```python
from build123d import *

# Parameters (mm, degrees)
SKETCH1_W           = 165
SKETCH1_H           = 330
BOSS_EXTRUDE1_DEPTH = 4
SKETCH2_R           = 37.5
CUT_EXTRUDE1_DEPTH  = 202.285866369
SKETCH4_W           = 8
SKETCH4_H           = 300
CUT_EXTRUDE3_DEPTH  = 202.285866369
SKETCH3_W           = 4
SKETCH3_H           = 20
CUT_EXTRUDE2_DEPTH  = 202.285866369
SKETCH5_W           = 8
SKETCH5_H           = 30
CUT_EXTRUDE4_DEPTH  = 202.285866369
SKETCH6_R           = 2
CUT_EXTRUDE5_DEPTH  = 198.838317825
SKETCH7_R           = 2
CUT_EXTRUDE6_DEPTH  = 198.838317825
SKETCH8_W           = 153
SKETCH8_H           = 20
CUT_EXTRUDE7_DEPTH  = 198.838317825


with BuildPart() as part:
    # Sketch1 → Boss-Extrude1 (new body)
    with BuildSketch(Plane.XY):
        with Locations((7.5, -15)):
            Rectangle(SKETCH1_W, SKETCH1_H)
    extrude(amount=BOSS_EXTRUDE1_DEPTH)

    # Sketch2 → Cut-Extrude1 (cut, through all)
    with BuildSketch(Plane.XY.offset(4)):
        with Locations((38, -159)):
            Circle(SKETCH2_R)
    extrude(amount=-CUT_EXTRUDE1_DEPTH, mode=Mode.SUBTRACT)

    # Sketch4 → Cut-Extrude3 (cut, through all)
    with BuildSketch(Plane(origin=(0, 0, 0), x_dir=(-1, 0, 0), z_dir=(0, 0, -1))):
        with Locations((-86, 0)):
            Rectangle(SKETCH4_W, SKETCH4_H)
    extrude(amount=-CUT_EXTRUDE3_DEPTH, mode=Mode.SUBTRACT)

    # Sketch3 → Cut-Extrude2 (cut, through all)
    with BuildSketch(Plane(origin=(0, 0, 0), x_dir=(-1, 0, 0), z_dir=(0, 0, -1))):
        with Locations((-80, 140)):
            Rectangle(SKETCH3_W, SKETCH3_H)
        with Locations((-80, 50)):
            Rectangle(SKETCH3_W, SKETCH3_H)
        with Locations((-80, -40)):
            Rectangle(SKETCH3_W, SKETCH3_H)
        with Locations((-80, -130)):
            Rectangle(SKETCH3_W, SKETCH3_H)
    extrude(amount=-CUT_EXTRUDE2_DEPTH, mode=Mode.SUBTRACT)

    # Sketch5 → Cut-Extrude4 (cut, through all)
    with BuildSketch(Plane.XY.offset(4)):
        with Locations((86, -165)):
            Rectangle(SKETCH5_W, SKETCH5_H)
    extrude(amount=-CUT_EXTRUDE4_DEPTH, mode=Mode.SUBTRACT)

    # Sketch6 → Cut-Extrude5 (cut, through all)
    with BuildSketch(Plane(origin=(0, 0, 0), x_dir=(-1, 0, 0), z_dir=(0, 0, -1))):
        with Locations((18, 120)):
            Circle(SKETCH6_R)
        with Locations((54, 120)):
            Circle(SKETCH6_R)
        with Locations((18, 68)):
            Circle(SKETCH6_R)
        with Locations((54, 68)):
            Circle(SKETCH6_R)
    extrude(amount=-CUT_EXTRUDE5_DEPTH, mode=Mode.SUBTRACT)

    # Sketch7 → Cut-Extrude6 (cut, through all)
    with BuildSketch(Plane.XY.offset(4)):
        with Locations((-65, 140)):
            Circle(SKETCH7_R)
        with Locations((-65, -10)):
            Circle(SKETCH7_R)
        with Locations((-65, -160)):
            Circle(SKETCH7_R)
    extrude(amount=-CUT_EXTRUDE6_DEPTH, mode=Mode.SUBTRACT)

    # Sketch8 → Cut-Extrude7 (cut, through all)
    with BuildSketch(Plane(origin=(0, 0, 0), x_dir=(-1, 0, 0), z_dir=(0, 0, -1))):
        with Locations((-1.5, 140)):
            Rectangle(SKETCH8_W, SKETCH8_H)
    extrude(amount=-CUT_EXTRUDE7_DEPTH, mode=Mode.SUBTRACT)


solid = part.part
```
For this review, take the finished solid that the model builds, in its own axes (mm). Give positions to 0.01 mm unless a question says otherwise; leave off trailing zeros. Write each loop counter-clockwise with the first axis right and the second up, starting at its lowest first coordinate (ties: lowest second). Pieces come first, ordered by that corner, then holes. Notation, with made-up numbers: M 8,-28 L 56,-28 A23 ccw 56,-3 Z; hole C -25.75,-13.75 d4. An arc over 180 degrees is marked long. Answer as CSV lines item,"result".
1. Consider section A-A, the plane z = 2.6. Write out the cut boundary in (x, y).
Findings:
outline,"M -75,-180 L 6.93,-180 A37.5 cw long 69.07,-180 L 82,-180 L 82,-140 L 78,-140 L 78,-120 L 82,-120 L 82,-50 L 78,-50 L 78,-30 L 82,-30 L 82,40 L 78,40 L 78,60 L 82,60 L 82,130 L -75,130 Z; hole C -65,-160 d4; hole C -65,-10 d4; hole C -54,68 d4; hole C -54,120 d4; hole C -18,68 d4; hole C -18,120 d4"
2. Consider section B-B, the plane y = -136. Write out the cut boundary in (x, z).
Findings:
outline,"M -75,0 L 8.38,0 L 8.38,4 L -75,4 Z; M 67.62,0 L 78,0 L 78,4 L 67.62,4 Z"
3. Draft analysis for pull direction Y (two halves, no side actions). For faces 1 (the flat face through (2, -23, 0)), 2 (the cylindrical face through (39.137, -121.517, 2.028)), state which applies: +Y half, -Y half, draft (parallel to the pull), parting line (faces both ways), or undercut.
Findings:
face 1,"draft"
face 2,"undercut"
4. Wall thickness on line 1 (Y direction, x = -18, z = 1.9); line 2 (Y direction, x = -65, z = 2.1); line 3 (X direction, y = -159, z = 3.05): over which ranges is each line inside the solid? List them lowest first.
Findings:
line 1,"y = -180 to 66, 70 to 118, 122 to 130"
line 2,"y = -180 to -162, -158 to -12, -8 to 130"
line 3,"x = -75 to -66.73, -63.27 to 0.5, 75.5 to 82"
5. Consider section D-D, the plane y = 48.5. Write out the cut boundary in (x, z), then the cut area to 3 significant figures.
Findings:
outline,"M -75,0 L 78,0 L 78,4 L -75,4 Z"
area,"612 mm2"
6. For pin 1 (2 mm diameter, centred on y = -36.5, z = 1.5, fed in from +X); pin 2 (1 mm diameter, centred on x = 56.5, z = 1.5, fed in from -Y), all flat-tipped, find the tip position at first contact; note any pin that passes through.
Findings:
pin 1,"stops at x = 78"
pin 2,"stops at y = -126.67"
7. Consider section C-C, the plane x = 38. Write out the cut boundary in (y, z).
Findings:
outline,"M -121.5,0 L 130,0 L 130,4 L -121.5,4 Z"
